Verification items for this drawing (mm, ordinates from the low corner). A direction names the side the tool comes from. Coordinates: 2 decimals unless noted, no trailing zeros. Order: outer loops, then holes, each group sorted by start corner. A loop starts at its lowest first (then second) coordinate and runs counter-clockwise, first axis right, second up. Notation, with made-up numbers: M -6,39.25 L 15,39.25 A19 cw 15,43.25 Z; hole C -3.5,78.25 d8. An arc over 180 degrees is marked long. Write item = value, one per line.
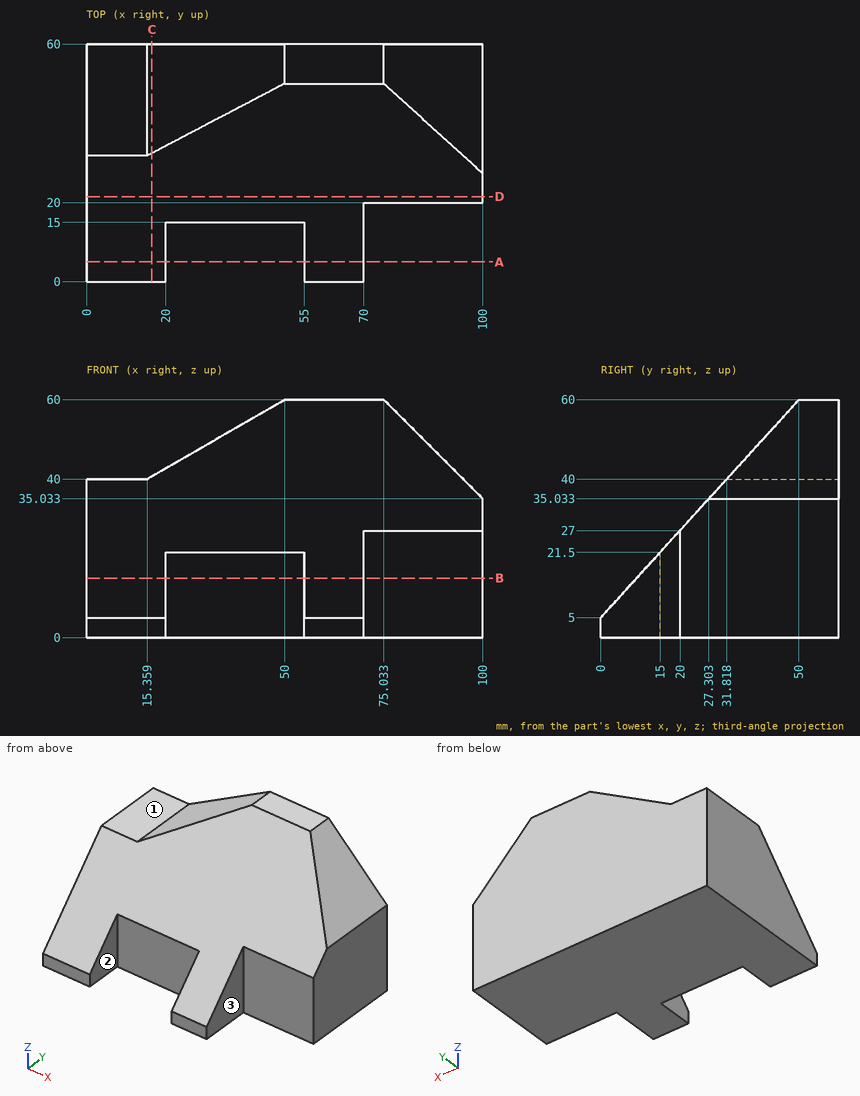
Item 1: Sectioned sample at B-B, the plane z = 15. Enter the section's corners in (x, y), then the cut area to 3 significant figures.
Report:
outline = M 0,9.09 L 20,9.09 L 20,15 L 55,15 L 55,9.09 L 70,9.09 L 70,20 L 100,20 L 100,60 L 0,60 Z
area = 4,560 mm^2
Item 2: Sectioned sample at A-A, the plane y = 5. Enter the section's corners in (x, z).
Report:
outline = M 0,0 L 20,0 L 20,10.5 L 0,10.5 Z; M 55,0 L 70,0 L 70,10.5 L 55,10.5 Z
Item 3: Sectioned sample at C-C, the plane x = 16.5. Enter the section's corners in (y, z), then the cut area to 3 significant figures.
Report:
outline = M 0,0 L 60,0 L 60,40.66 L 32.42,40.66 L 0,5 Z
area = 1,860 mm^2
Item 4: Scan lines: L1, parallel to Y at x = 23.5, z = 18; L2, parallel to Z at x = 12, y = 55; L3, parallel to Y at x = 73, z = 8. Record each from-to range of solid material in increasing order. Write a range as from..to.
Report:
L1 = 15..60
L2 = 0..40
L3 = 20..60
Item 5: Gauge pin test, flat ends, axial feed: pin 1 (16.5 mm diameter, centred on y = 10, z = 6, fed in from +X); pin 2 (23.5 mm diameter, centred on x = 45, z = 15.5, fed in from -Y) (1 decimal); pin 3 (8 mm diameter, centred on x = 62.5, z = 19, fed in from -Y). Record the tip position at first contact, or that the pin passes through.
Report:
pin_1 = 70
pin_2 = 3.9
pin_3 = 9.09
Item 6: Tool access check on the marked faces 1, 2 and 3. Record the directions out of +Z, -Z, +X, -X, +Y, -Y that give a thin tool (end or side, any length) a straight path to the whole face; none if there is none.
Report:
face_1 = +Z, -X, +Y, -Y
face_2 = +Z, -Z, -Y
face_3 = +Z, -Z, +X, -Y
Item 7: Sectioned sample at D-D, the plane y = 21.5. Enter the section's corners in (x, z), then the cut area to 4 significant figures.
Report:
outline = M 0,0 L 100,0 L 100,28.65 L 0,28.65 Z
area = 2,865 mm^2
